Input: part model. Units: mm. Frame: model coordinates. A direction names the side the tool comes from. Coordinates: 2 decimals unless noted, no trailing zeros. Loops run counter-clockwise (first coordinate to the right, second up) from the corner with the lowest first, then second, coordinate; pieces in that order, holes last.
Item 1: Section B-B on y = -260. Return loops of the section in (x, z), and give its area (3 significant figures).
Item 2: Contact query for flat-ended pins moving along their axis: P1, Ø11, axis at x = 369.5, z = 198, coming from the +Y side; P2, Ø6, axis at x = 18.47, y = -260, coming from the +Z side. Output: stop coordinate, or through.
Item 3: Section C-C on x = 198.5. Return loops of the section in (y, z), and give its area (3 significant figures).
Item 4: Section A-A on z = 244.5. Return loops of the section in (x, y), and give its area (3 significant figures).
Item 5: Pull-direction query (X, two-part tool) for faces 4 (the cylindrical face through (2.85, -316.99, 136.75)), 5 (the flat face through (217, -158, 0)), 6 (the cylindrical face through (436.99, -157.9, 2.85)), 7 (the flat face through (48.471, -163, 152)); classes: released by +X, released by -X, zero draft, split by the parting line, or undercut.
Item 6: Ray query, line 1 along X through (y, z) = (-260, 252); line 2 along Y through (x, z) = (103, 148.5); line 3 along X through (y, z) = (-261, 232). Return the intervals inside material, ascending.
Item 7: Section D-D on z = 200. Return loops of the section in (x, y), and give its area (3 significant figures).
Item 8: Reachability of faces 1 (the flat face through (222, -41.867, 152)), 2 (the flat face through (440, -162, 133)), 3 (the cylindrical face through (374.957, -4.93, 199.349)) from +Z, -Z, +X, -X, +Y, -Y: full face, straight path, thin tool, end or side. Return the list, or none.
```python
from build123d import *

# Parameters (mm, degrees)
SKETCH_1_W          = 440
SKETCH_1_H          = 320
EXTRUDE_1_DEPTH     = 260
SKETCH_6_W          = 351.529236831
SKETCH_6_H          = 238.132708821
CUT_EXTRUDE_1_DEPTH = 220
FILLET_1_R          = 10
SKETCH_7_R          = 5
CUT_EXTRUDE_2_DEPTH = 10
SKETCH_8_R          = 5
CUT_EXTRUDE_3_DEPTH = 10


with BuildPart() as part:
    # 草图1 → 凸台-拉伸1 (new body)
    with BuildSketch(Plane.XY):
        with Locations((220, -160)):
            Rectangle(SKETCH_1_W, SKETCH_1_H)
    extrude(amount=EXTRUDE_1_DEPTH)

    # 草图6 → 切除-拉伸1 (cut)
    with BuildSketch(Plane.XY.offset(260)):
        with Locations((224.235381585, -160.93364559)):
            Rectangle(SKETCH_6_W, SKETCH_6_H)
    extrude(amount=-CUT_EXTRUDE_1_DEPTH, mode=Mode.SUBTRACT)

    # 圆角1
    fillet_1_edges = [part.edges().sort_by_distance(p)[0] for p in [
        (220, 0, 0),
        (440, -160, 0),
        (220, -320, 0),
        (0, -160, 0),
        (0, 0, 130),
        (440, 0, 130),
        (440, -320, 130),
        (0, -320, 130),
    ]]
    fillet(fillet_1_edges, radius=FILLET_1_R)

    # 草图7 → 切除-拉伸2 (cut)
    with BuildSketch(Plane.XY.offset(260)):
        with Locations((18.470763169, -60)):
            Circle(SKETCH_7_R)
        with Locations((18.470763169, -260)):
            Circle(SKETCH_7_R)
    extrude(amount=-CUT_EXTRUDE_2_DEPTH, mode=Mode.SUBTRACT)

    # 草图8 → 切除-拉伸3 (cut)
    with BuildSketch(Plane(origin=(0, 0, 0), x_dir=(1, 0, 0), z_dir=(0, 1, 0))):
        with Locations(Location((370, -200, 0), (0, 0, 270))):
            Circle(SKETCH_8_R)
    extrude(amount=-CUT_EXTRUDE_3_DEPTH, mode=Mode.SUBTRACT)


solid = part.part
```
Results found:
1. outline: (0, 10) arc R10 ccw to (10, 0) - (430, 0) arc R10 ccw to (440, 10) - (440, 260) - (400, 260) - (400, 40) - (48.47, 40) - (48.47, 260) - (23.47, 260) - (23.47, 250) - (13.47, 250) - (13.47, 260) - (0, 260) - close
1. area: 36,900 mm2
2. P1: stops at y = 0
2. P2: stops at z = 250
3. outline: (-320, 10) arc R10 ccw to (-310, 0) - (-10, 0) arc R10 ccw to (0, 10) - (0, 260) - (-41.87, 260) - (-41.87, 40) - (-280, 40) - (-280, 260) - (-320, 260) - close
3. area: 30,800 mm2
4. outline: (0, -310) arc R10 ccw to (10, -320) - (430, -320) arc R10 ccw to (440, -310) - (440, -10) arc R10 ccw to (430, 0) - (10, 0) arc R10 ccw to (0, -10) - close; hole (48.47, -280) - (400, -280) - (400, -41.87) - (48.47, -41.87) - close
4. area: 57,000 mm2
5. face 4: released by -X
5. face 5: zero draft
5. face 6: released by +X
5. face 7: undercut
6. line 1: x = 0 to 13.47, 23.47 to 48.47, 400 to 440
6. line 2: y = -320 to -280, -41.87 to 0
6. line 3: x = 0 to 48.47, 400 to 440
7. outline: (0, -310) arc R10 ccw to (10, -320) - (430, -320) arc R10 ccw to (440, -310) - (440, -10) arc R10 ccw to (430, 0) - (375, 0) - (375, -10) - (365, -10) - (365, 0) - (10, 0) arc R10 ccw to (0, -10) - close; hole (48.47, -280) - (400, -280) - (400, -41.87) - (48.47, -41.87) - close
7. area: 56,900 mm2
8. face 1: +Z
8. face 2: +Z, -Z, +X, +Y, -Y
8. face 3: +Y
